```python
from build123d import *

# Parameters (mm, degrees)
F0_R     = 15
F0_R_2   = 8.75
F1_DEPTH = 21
F0_R_3   = 20
F2_DEPTH = 3
F0_R_4   = 42
F0_R_5   = 4
F3_DEPTH = 6
F4_DEPTH = 6
F0_R_6   = 5
F5_DEPTH = 3
F6_DEPTH = 3
F7_DEPTH = 1
F8_SIZE  = 3.74999


# Not quite as in the source:
# - a fillet or chamfer is up to 0.001 mm smaller than in the source, because OpenCascade refuses the exact size


with BuildPart() as f1:
    # F0 (on Top) → F1 (new body)
    with BuildSketch(Plane.XY):
        Circle(F0_R)
        Circle(F0_R_2, mode=Mode.SUBTRACT)
    extrude(amount=F1_DEPTH)

    # F0 (on Top) → F2 (join)
    with BuildSketch(Plane.XY):
        Circle(F0_R_3)
        Circle(F0_R, mode=Mode.SUBTRACT)
    extrude(amount=-F2_DEPTH)

    # F0 (on Top) → F3 (join)
    with BuildSketch(Plane.XY):
        Circle(F0_R_4)
        with Locations((-24.7487373415, -24.7487373415)):
            Circle(F0_R_5, mode=Mode.SUBTRACT)
        with Locations((0, -35)):
            Circle(F0_R_5, mode=Mode.SUBTRACT)
        with Locations((24.7487373415, -24.7487373415)):
            Circle(F0_R_5, mode=Mode.SUBTRACT)
        with Locations((-35, 0)):
            Circle(F0_R_5, mode=Mode.SUBTRACT)
        with Locations((-24.7487373415, 24.7487373415)):
            Circle(F0_R_5, mode=Mode.SUBTRACT)
        Circle(F0_R_3, mode=Mode.SUBTRACT)
        with Locations((35, 0)):
            Circle(F0_R_5, mode=Mode.SUBTRACT)
        with Locations((0, 35)):
            Circle(F0_R_5, mode=Mode.SUBTRACT)
        with Locations((24.7487373415, 24.7487373415)):
            Circle(F0_R_5, mode=Mode.SUBTRACT)
    extrude(amount=F3_DEPTH)

    # F0 (on Top) → F4 (join)
    with BuildSketch(Plane.XY):
        Circle(F0_R_3)
        Circle(F0_R, mode=Mode.SUBTRACT)
    extrude(amount=F4_DEPTH)

    # F0 (on Top) → F5 (join)
    with BuildSketch(Plane.XY):
        Circle(F0_R_2)
        Circle(F0_R_6, mode=Mode.SUBTRACT)
    extrude(amount=-F5_DEPTH)

    # F0 (on Top) → F6 (join)
    with BuildSketch(Plane.XY):
        Circle(F0_R)
        Circle(F0_R_2, mode=Mode.SUBTRACT)
    extrude(amount=-F6_DEPTH)

    # F0 (on Top) → F7 (join)
    with BuildSketch(Plane.XY):
        Circle(F0_R_2)
        Circle(F0_R_6, mode=Mode.SUBTRACT)
    extrude(amount=F7_DEPTH)

    # F8 (size 3.75 in the source; OpenCascade refuses exactly that, so slightly less here)
    f8_edges = [f1.edges().sort_by_distance(p)[0] for p in [
        (-8.75, 0, 1),
    ]]
    chamfer(f8_edges, length=F8_SIZE)


solid = f1.part
```
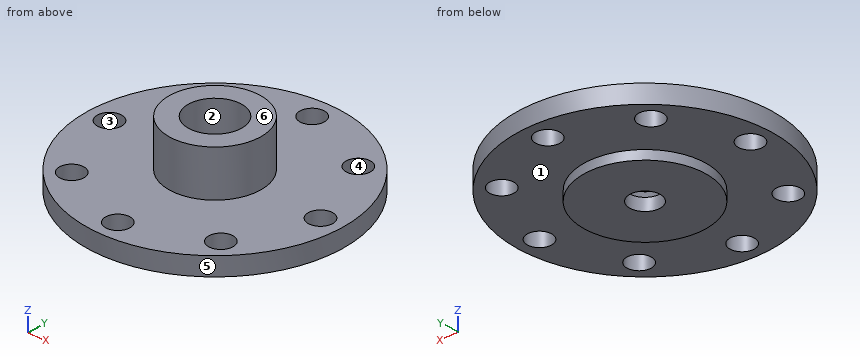
Model file for the job. Use its own axes, mm. Face numbers are marked on the shaded views. A direction names the side the tool comes from. Coordinates: 2 decimals unless noted, no trailing zeros. Loops run counter-clockwise (first coordinate to the right, second up) from the corner with the lowest first, then second, coordinate; pieces in that order, holes last. Notation, with made-up numbers: (18.5, -4.5) - (30.5, -4.5) arc R36 ccw to (30.5, 31.5) - close; hole circle Ø6 at (-26.75, 78.25). An arc over 180 degrees is marked (long way). Answer as a JSON object with one key per item and string values. Group by question number.
(1) Cut at D-D (y = 35). Give the cut face in (x, z), then the cut area to 3 significant figures.
(2) Flat gauge pins, fed straight in: pin 1 (13 mm diameter, centred on x = -24.75, y = 24.75, fed in from +Z); pin 2 (11 mm diameter, centred on x = -2.5, y = 2, fed in from +Z); pin 3 (6 mm diameter, centred on y = 14, z = 13, fed in from +X). Where does each tip first touch, or does it go through?
(3) Cut at A-A (x = 0). State how many separate pieces and enclosed holes the cut face has, then the cut area to 3 significant figures.
(4) Two-plate mould, pull along Y, no slides. Class the marked faces 4, 5 and 6: released by +Y, released by -Y, zero draft, split by the parting line, or undercut.
(5) Tool access for the marked faces 1, 2 and 3: list every direction of +Z, -Z, +X, -X, +Y, -Y with a clear straight run to the whole face (end or side of a thin tool).
(6) Probe line 1 along X through (y, z) = (28, 0.25); line 2 along Z through (x, y) = (-21, 7); line 3 along X through (y, z) = (7, 12.5). List the from-to ranges inside material, lowest first.
(7) Cut at C-C (x = -32). Give the cut face in (y, z), then the cut area to 3 significant figures.
Geometry says:
{
 "1": {"outline": "(-23.22, 0) - (-4, 0) - (-4, 6) - (-23.22, 6) - close; (4, 0) - (23.22, 0) - (23.22, 6) - (4, 6) - close", "area": "231 mm^2"},
 "2": {"pin 1": "stops at z = 6", "pin 2": "stops at z = 4.7", "pin 3": "stops at x = 10.2"},
 "3": {"separate pieces": "4", "enclosed holes": "0", "area": "602 mm^2"},
 "4": {"face 4": "undercut", "face 5": "split by the parting line", "face 6": "zero draft"},
 "5": {"face 1": "-Z", "face 2": "+Z", "face 3": "+Z, -Z"},
 "6": {"line 1": "x = -31.3 to -27.08, -22.42 to 22.42, 27.08 to 31.3", "line 2": "z = 0 to 6", "line 3": "x = -13.27 to -5.25, 5.25 to 13.27"},
 "7": {"outline": "(-27.2, 0) - (-2.65, 0) - (-2.65, 6) - (-27.2, 6) - close; (2.65, 0) - (27.2, 0) - (27.2, 6) - (2.65, 6) - close", "area": "295 mm^2"}
}
